Geometry check sheet. Reference: the model listing, model coordinates, mm. A direction names the side the tool comes from. Coordinates: 2 decimals unless noted, no trailing zeros. Write each loop counter-clockwise with the first axis right and the second up, starting at its lowest first coordinate (ties: lowest second). Pieces come first, ordered by that corner, then holes. Notation, with made-up numbers: (84.5, 35.5) - (103.5, 35.5) arc R18 ccw to (103.5, 64.5) - close; hole circle Ø3 at (16.5, 66.5). An arc over 180 degrees is marked (long way). Answer as a JSON object with one key per item and string values. Group by question number.
from build123d import *

# Parameters (mm, degrees)
F0_R           = 3.175
F1_DEPTH       = 4.7752
F3_DEPTH       = 7.9248
F4_SIZE        = 6.35
F6_D           = 3.4544
F6_START       = 1.4605
F6_CBORE_D     = 5.461
F6_CBORE_DEPTH = 11.0998
F8_D           = 3.4544
F8_DEPTH       = 5.08
F8_TIP         = 1.0378064612
F9_T4_DEPTH    = 4.7752
F9_S5_R        = 2.7305
F9_T6_DEPTH    = 4
F9_T10_DEPTH   = 4.7752
F9_S11_R       = 2.7305
F9_T12_DEPTH   = 4


# Not quite as in the source:
# - a fillet or chamfer that OpenCascade refuses, or shapes differently, is made with other operations: its cross-section is extruded or revolved along the edge and cut away or added


with BuildPart() as f1:
    # F0 (on Front) → F1 (new body)
    with BuildSketch(Plane.XZ):
        with BuildLine():
            ThreePointArc((-8.2574477487, 44.9918270709), (-7.0896388893, 46.4434074028), (-5.3086, 46.99))
            Line((-5.3086, 46.99), (5.3086, 46.99))
            ThreePointArc((5.3086, 46.99), (7.0896388893, 46.4434074028), (8.2574477487, 44.9918270709))
            Line((8.2574477487, 44.9918270709), (26.2128, 0))
            Line((26.2128, 0), (38.1, 0))
            Line((38.1, 0), (38.1, 20.6248))
            Line((38.1, 20.6248), (27.6356818802, 20.6248))
            Line((27.6356818802, 20.6248), (11.2650625427, 61.6456646408))
            ThreePointArc((11.2650625427, 61.6456646408), (0, 69.2789997383), (-11.2650625427, 61.6456646408))
            Line((-11.2650625427, 61.6456646408), (-27.6356818802, 20.6248))
            Line((-27.6356818802, 20.6248), (-38.1, 20.6248))
            Line((-38.1, 20.6248), (-38.1, 0))
            Line((-38.1, 0), (-26.2128, 0))
            Line((-26.2128, 0), (-8.2574477487, 44.9918270709))
        make_face()
        with Locations((0, 57.15)):
            Circle(F0_R, mode=Mode.SUBTRACT)
    extrude(amount=F1_DEPTH)

    # F2 (on face) → F3 (join)
    with BuildSketch(Plane.XZ.offset(4.7752)):
        Polygon((-27.6356818802, 20.6248), (-38.1, 20.6248), (-38.1, 0), (-26.2128, 0), (-26.2128, 20.6248), align=None)
        Polygon((38.1, 20.6248), (27.6356818802, 20.6248), (26.2128, 20.6248), (26.2128, 0), (38.1, 0), align=None)
    extrude(amount=F3_DEPTH)

    # F4
    f4_edges = [f1.edges().sort_by_distance(p)[0] for p in [
        (38.1, -6.35, 20.6248),
        (-38.1, -6.35, 20.6248),
    ]]
    chamfer(f4_edges, length=F4_SIZE)

    # F6 (through all)
    # its depths count from where the whole tool has entered the part; down to there all is cleared
    with Locations(Plane.XY.offset(20.6248).offset(-F6_START)):
        with Locations((-30.48, -6.35), (30.48, -6.35)):
            CounterBoreHole(F6_D / 2, F6_CBORE_D / 2, F6_CBORE_DEPTH)

    # F8
    with Locations(Plane(origin=(0, 0, 0), x_dir=(-1, 0, 0), z_dir=(0, 1, 0))):
        with Locations((-24.0792, 18.288), (24.0792, 18.288)):
            Hole(F8_D / 2, depth=F8_DEPTH)
            with Locations((0, 0, -(F8_DEPTH + F8_TIP / 2))):  # 118° drill point
                Cone(0, F8_D / 2, F8_TIP, mode=Mode.SUBTRACT)

    # F9: fillet of radius 3.175 on 2 edges, made by hand


with BuildPart() as f9_tool2:
    # F9_s3 → F9_t4 (new body)
    with BuildSketch(Plane.XZ):
        with BuildLine():
            ThreePointArc((-29.7870981589, 20.6248), (-28.0060592696, 21.1713925972), (-26.8382504101, 22.6229729291))
            Line((-26.8382504101, 22.6229729291), (-27.6356818802, 20.6248))
            Line((-27.6356818802, 20.6248), (-29.7870981589, 20.6248))
        make_face()
    extrude(amount=F9_T4_DEPTH)

    # F9_s5 → F9_t6 (cut, symmetric)
    with BuildSketch(Plane.XY.offset(21.6)):
        with Locations((-30.48, -6.35)):
            Circle(F9_S5_R)
    extrude(amount=F9_T6_DEPTH, both=True, mode=Mode.SUBTRACT)


with BuildPart() as f1_1:
    add(f1.part)

    # F9_t1: union F9_tool2
    add(f9_tool2.part)


with BuildPart() as f9_tool8:
    # F9_s9 → F9_t10 (new body)
    with BuildSketch(Plane.XZ):
        with BuildLine():
            ThreePointArc((26.8382504101, 22.6229729291), (28.0060592696, 21.1713925972), (29.7870981589, 20.6248))
            Line((29.7870981589, 20.6248), (27.6356818802, 20.6248))
            Line((27.6356818802, 20.6248), (26.8382504101, 22.6229729291))
        make_face()
    extrude(amount=F9_T10_DEPTH)

    # F9_s11 → F9_t12 (cut, symmetric)
    with BuildSketch(Plane.XY.offset(21.6)):
        with Locations((30.48, -6.35)):
            Circle(F9_S11_R)
    extrude(amount=F9_T12_DEPTH, both=True, mode=Mode.SUBTRACT)


with BuildPart() as f1_2:
    add(f1_1.part)

    # F9_t7: union F9_tool8
    add(f9_tool8.part)


solid = f1_2.part
(1) Draft check along Y on faces 5 (the face through (31, -2, 20.625)), 6 (the face through (-32, -5, 8.065)), 7 (the face through (-27.876, -5.53, 14.634)), 8 (the face through (11.5, 0, 37.4)). Enter one of: +Y half, -Y half, draft (parallel to the pull), parting line (faces both ways), or undercut.
(2) Material ranges on L1, parallel to X at y = -8.75, z = 8; L2, parallel to X at y = -2, z = 21; L3, parallel to X at y = -6, z = 11, recorded low to high. Write a range as [from, to].
(3) Gauge pin test, flat ends, axial feed: pin 1 (5 mm diameter, centred on y = -4.5, z = 26, fed in from +X); pin 2 (4.5 mm diameter, centred on x = -30.48, y = -6.35, fed in from -Z); pin 3 (3 mm diameter, centred on x = -30.48, y = -6.35, fed in from -Z); pin 4 (10 mm diameter, centred on x = 0, z = 57.15, fed in from -Y). Record the tip position at first contact, or that the pin passes through.
(4) Section check B-B (z = 11.5). Record the cut outline in (x, y), and give its area (3 significant figures).
(5) Section check C-C (y = -6.35). Record the cut outline in (x, z), and give its area (3 significant figures).
(6) Section check A-A (x = 0). Record the cut outline in (y, z) (3 decimals).
(7) Section check D-D (y = -2). Record the cut outline in (x, z) (3 decimals).
(8) Set-up check for faces 1 (the face through (26.213, -9, 10)), 2 (the face through (-38.1, -6, 7)), 3 (the face through (28, -10, 20.625)), 4 (the face through (-7.11, -2.35, 46.43)): record each of +Z, -Z, +X, -X, +Y, -Y from which the full face is reachable in a straight line by a thin tool's end or side.
Conclusion:
{
 "1": {"face 5": "draft", "face 6": "undercut", "face 7": "undercut", "face 8": "+Y half"},
 "2": {"L1": "x = [-38.1, -26.21], [26.21, 38.1]", "L2": "x = [-28.29, -17.83], [17.83, 28.29]", "L3": "x = [-38.1, -33.19], [-27.77, -26.21], [26.21, 27.77], [33.19, 38.1]"},
 "3": {"pin 1": "stops at x = 26.49", "pin 2": "stops at z = 0", "pin 3": "passes through", "pin 4": "stops at y = -4.78"},
 "4": {"outline": "(-38.1, -12.7) - (-26.21, -12.7) - (-26.21, -4.78) - (-21.62, -4.78) - (-21.62, 0) - (-38.1, 0) - close; (21.62, -4.78) - (26.21, -4.78) - (26.21, -12.7) - (38.1, -12.7) - (38.1, 0) - (21.62, 0) - close; hole circle Ø5.46 at (-30.48, -6.35); hole circle Ø5.46 at (30.48, -6.35)", "area": "299 mm^2"},
 "5": {"outline": "(-38.1, 0) - (-32.21, 0) - (-32.21, 8.06) - (-33.21, 8.06) - (-33.21, 19.16) - (-38.1, 14.27) - close; (-28.75, 0) - (-26.21, 0) - (-26.21, 20.62) - (-27.75, 20.62) - (-27.75, 8.06) - (-28.75, 8.06) - close; (26.21, 0) - (28.75, 0) - (28.75, 8.06) - (27.75, 8.06) - (27.75, 20.62) - (26.21, 20.62) - close; (32.21, 0) - (38.1, 0) - (38.1, 14.27) - (33.21, 19.16) - (33.21, 8.06) - (32.21, 8.06) - close", "area": "259 mm^2"},
 "6": {"outline": "(-4.775, 46.99) - (0, 46.99) - (0, 53.975) - (-4.775, 53.975) - close; (-4.775, 60.325) - (0, 60.325) - (0, 69.279) - (-4.775, 69.279) - close"},
 "7": {"outline": "(-38.1, 0) - (-26.213, 0) - (-8.257, 44.992) arc R3.175 cw to (-5.309, 46.99) - (5.309, 46.99) arc R3.175 cw to (8.257, 44.992) - (26.213, 0) - (38.1, 0) - (38.1, 14.275) - (31.75, 20.625) - (29.787, 20.625) arc R3.175 cw to (26.838, 22.623) - (11.265, 61.646) arc R12.129 ccw to (-11.265, 61.646) - (-26.838, 22.623) arc R3.175 cw to (-29.787, 20.625) - (-31.75, 20.625) - (-38.1, 14.275) - close; hole circle Ø3.454 at (-24.079, 18.288); hole circle Ø6.35 at (0, 57.15); hole circle Ø3.454 at (24.079, 18.288)"},
 "8": {"face 1": "+Z, -Z, -Y", "face 2": "+Z, -Z, -X, +Y, -Y", "face 3": "+Z, +X, -X, -Y", "face 4": "-Z, +Y, -Y"}
}
